```python
from build123d import *

# Parameters (mm, degrees)
SKETCH074_W     = 73.4
SKETCH074_H     = 71.4
PAD024_DEPTH    = 10
SKETCH075_W     = 71
SKETCH075_H     = 69
POCKET045_DEPTH = 9.2
SKETCH076_R     = 3.3
POCKET046_DEPTH = 1.2
SKETCH077_R     = 2.75
PAD025_DEPTH    = 9.8
SKETCH078_R     = 1.55
POCKET047_DEPTH = 10
SKETCH079_R     = 2.2
POCKET048_DEPTH = 2.8
FILLET001_R     = 2
FILLET002_R     = 2
FILLET003_R     = 2


with BuildPart() as part:
    # Sketch074 (on XY_Plane416 of Origin554) → Pad024 (new body)
    with BuildSketch(Plane.XY):
        with Locations((0, 26.5)):
            Rectangle(SKETCH074_W, SKETCH074_H)
    extrude(amount=-PAD024_DEPTH)

    # Sketch075 (on XY_Plane416 of Origin554) → Pocket045 (cut)
    with BuildSketch(Plane.XY):
        with Locations((0, 26.5)):
            Rectangle(SKETCH075_W, SKETCH075_H)
    extrude(amount=-POCKET045_DEPTH, mode=Mode.SUBTRACT)

    # Sketch076 (on XZ_Plane416 of Origin554) → Pocket046 (cut)
    with BuildSketch(Plane.XZ.offset(-62.2)):
        with Locations((18.35, -5)):
            Circle(SKETCH076_R)
        with Locations((0, -5)):
            Circle(SKETCH076_R)
        with Locations((-18.35, -5)):
            Circle(SKETCH076_R)
    extrude(amount=POCKET046_DEPTH, mode=Mode.SUBTRACT)

    # Sketch077 (on XY_Plane416 of Origin554) → Pad025 (join)
    with BuildSketch(Plane.XY.offset(-0.2)):
        with Locations((-32, 55.5)):
            Circle(SKETCH077_R)
        with Locations((32, 55.5)):
            Circle(SKETCH077_R)
        with Locations((32, -4.5)):
            Circle(SKETCH077_R)
        with Locations((-32, -4.5)):
            Circle(SKETCH077_R)
    extrude(amount=-PAD025_DEPTH)

    # Sketch078 (on XY_Plane416 of Origin554) → Pocket047 (cut)
    with BuildSketch(Plane.XY):
        with Locations((32, 55.5)):
            Circle(SKETCH078_R)
        with Locations((-32, 55.5)):
            Circle(SKETCH078_R)
        with Locations((-32, -4.5)):
            Circle(SKETCH078_R)
        with Locations((32, -4.5)):
            Circle(SKETCH078_R)
    extrude(amount=-POCKET047_DEPTH, mode=Mode.SUBTRACT)

    # Sketch079 (on XY_Plane416 of Origin554) → Pocket048 (cut)
    with BuildSketch(Plane.XY.offset(-7.2)):
        with Locations((-32, 55.5)):
            Circle(SKETCH079_R)
        with Locations((32, 55.5)):
            Circle(SKETCH079_R)
        with Locations((32, -4.5)):
            Circle(SKETCH079_R)
        with Locations((-32, -4.5)):
            Circle(SKETCH079_R)
    extrude(amount=-POCKET048_DEPTH, mode=Mode.SUBTRACT)

    # Fillet001
    fillet001_edges = [part.edges().sort_by_distance(p)[0] for p in [
        (0, -9.2, -10),
    ]]
    fillet(fillet001_edges, radius=FILLET001_R)

    # Fillet002
    fillet002_edges = [part.edges().sort_by_distance(p)[0] for p in [
        (36.7, 27.5, -10),
    ]]
    fillet(fillet002_edges, radius=FILLET002_R)

    # Fillet003
    fillet003_edges = [part.edges().sort_by_distance(p)[0] for p in [
        (-36.7, 27.5, -10),
    ]]
    fillet(fillet003_edges, radius=FILLET003_R)


with BuildPart() as part_1:
    # Body005 placement: moved
    add(part.part.moved(Location((0, 0, -13.7))))


solid = part_1.part
```
Geometry check sheet. Reference: the model listing, model coordinates, mm. A direction names the side the tool comes from. Coordinates: 2 decimals unless noted, no trailing zeros. Write each loop counter-clockwise with the first axis right and the second up, starting at its lowest first coordinate (ties: lowest second). Pieces come first, ordered by that corner, then holes. Notation, with made-up numbers: M -17,78.5 L -4,78.5 A27 ccw -4,115.5 Z; hole C 34,44 d11. An arc over 180 degrees is marked long. Use one line per item in the form item = value. Start each with the question number.
1) Section check D-D on x = 18.35. Enter the section's corners in (y, z), and give its area (3 significant figures).
2) Thickness scan on probe 1 along Y at (x, z) = (32, -21.65); probe 2 along Y at (x, z) = (32, -15.25); probe 3 along Y at (x, z) = (-6.5, -16.75). Record the ranges inside material, lowest first. Write a range as from..to.
3) Set-up check for faces 1 (the flat face through (0, 28, -23.7)), 2 (the flat face through (0, 27, -22.9)), 3 (the cylindrical face through (33.478, -4.034, -17.351)), 4 (the cylindrical face through (31.523, 53.352, -22.28)), 5 (the cylindrical face through (-2.43, 61.61, -16.47)): record each of +Z, -Z, +X, -X, +Y, -Y from which the full face is reachable in a straight line by a thin tool's end or side.
4) Release check for a two-part mould opening along Y. For faces 6 (the cylindrical face through (-36.13, 27.99, -23.1)), 7 (the flat face through (0, -9.2, -18)), 8 (the flat face through (31, 57, -20.9)) record: pulls with the +Y half, pulls with the -Y half, needs draft (parallel to the pull), parting line crosses it, or undercut.
5) Section check A-A on y = 55.5. State how many separate pieces and enclosed holes the cut face has, and give its area (3 significant figures).
6) Go/stop test with flat-tipped pins: pin 1 Ø2 at (x, y) = (-14, 9.5) entering from +Z; pin 2 Ø4 at (x, y) = (32, -4.5) entering from -Z; pin 3 Ø5.5 at (x, y) = (32, -4.5) entering from +Z; pin 4 Ø6 at (x, y) = (-33, -5.5) entering from +Z. Record where each tip stops, or that it passes through.
Responses:
q1.outline = M -9.2,-21.7 A2 ccw -7.2,-23.7 L 62.2,-23.7 L 62.2,-22 L 61,-22 L 61,-22.9 L -8,-22.9 L -8,-13.7 L -9.2,-13.7 Z; M 61,-15.4 L 62.2,-15.4 L 62.2,-13.7 L 61,-13.7 Z
q1.area = 70.4 mm2
q2.probe_1 = -9.2..-8, -7.25..-6.7, -2.3..-1.75, 52.75..53.3, 57.7..58.25, 61..62.2
q2.probe_2 = -9.2..-8, -7.25..-6.05, -2.95..-1.75, 52.75..53.95, 57.05..58.25, 61..62.2
q2.probe_3 = -9.2..-8, 61..62.2
q3.face_1 = -Z, +X, -X, +Y, -Y
q3.face_2 = +Z
q3.face_3 = +Z, -Z
q3.face_4 = -Z
q3.face_5 = +Y
q4.face_6 = needs draft
q4.face_7 = pulls with the -Y half
q4.face_8 = undercut
q5.separate_pieces = 3
q5.enclosed_holes = 0
q5.area = 110 mm2
q6.pin_1 = -22.9
q6.pin_2 = -20.9
q6.pin_3 = -13.9
q6.pin_4 = -13.7
